```python
from build123d import *

# Parameters (mm, degrees)
SKETCH1_W           = 3.047619048
SKETCH1_H           = 150
SKETCH1_W_2         = 38
SKETCH1_H_2         = 3
BOSS_EXTRUDE1_DEPTH = 15
FILLET1_R           = 10
SKETCH2_R           = 2.5
CUT_EXTRUDE1_DEPTH  = 61
SKETCH3_R           = 2.5
CUT_EXTRUDE2_DEPTH  = 55


with BuildPart() as part:
    # Sketch1 → Boss-Extrude1 (new, symmetric)
    with BuildSketch(Plane.XY):
        with Locations((-20.523809524, 25)):
            Rectangle(SKETCH1_W, SKETCH1_H)
        with Locations((20.523809524, 25)):
            Rectangle(SKETCH1_W, SKETCH1_H)
        with Locations((0, 74.5)):
            Rectangle(SKETCH1_W_2, SKETCH1_H_2)
        with Locations((0, -28.5)):
            Rectangle(SKETCH1_W_2, SKETCH1_H_2)
    extrude(amount=BOSS_EXTRUDE1_DEPTH, both=True)

    # Fillet1
    fillet1_edges = [part.edges().sort_by_distance(p)[0] for p in [
        (-20.523809524, -50, -15),
        (20.523809524, -50, -15),
        (20.523809524, -50, 15),
        (-20.523809524, -50, 15),
        (-20.523809524, 100, 15),
        (-20.523809524, 100, -15),
        (20.523809524, 100, -15),
        (20.523809524, 100, 15),
    ]]
    fillet(fillet1_edges, radius=FILLET1_R)

    # Sketch2 → Cut-Extrude1 (cut)
    with BuildSketch(Plane(origin=(22.047619048, 0, 0), x_dir=(0, 0, -1), z_dir=(1, 0, 0))):
        with Locations(Location((0, 41.439583657, 0), (0, 0, 90))):
            Circle(SKETCH2_R)
        with Locations(Location((0, -40.747770908, 0), (0, 0, 90))):
            Circle(SKETCH2_R)
    extrude(amount=-CUT_EXTRUDE1_DEPTH, mode=Mode.SUBTRACT)

    # Sketch3 → Cut-Extrude2 (cut)
    with BuildSketch(Plane(origin=(22.047619048, 0, 0), x_dir=(0, 0, -1), z_dir=(1, 0, 0))):
        with Locations(Location((0, 90.824457964, 0), (0, 0, 90))):
            Circle(SKETCH3_R)
    extrude(amount=-CUT_EXTRUDE2_DEPTH, mode=Mode.SUBTRACT)


solid = part.part
```
Build history of the part. All positions in model axes, mm. A direction names the side the tool comes from. Coordinates: 2 decimals unless noted, no trailing zeros. Order: outer loops, then holes, each group sorted by start corner. A loop starts at its lowest first (then second) coordinate and runs counter-clockwise, first axis right, second up. Notation, with made-up numbers: (-34, 29) -> (6, 29) arc R20 cw to (6, 42) -> close; hole circle Ø7 at (67, -23). An arc over 180 degrees is marked (long way). Answer in a Markdown table with one row per item. Add a question column.
Q1. Band-saw the part on A-A, the plane y = 53. List the corners of the cut face in (x, z), then the cut area to 3 significant figures.
Q2. Mould opens along X. For faces 4 (the face through (-20.5, 96.99, 12.15)), 5 (the face through (19, -38, 0)), 6 (the face through (-22.048, 24, 0)), 7 (the face through (0, -30, 0)) say: +X half, -X half, draft (parallel to the pull), parting line (faces both ways), or undercut.
Q3. Band-saw the part on C-C, the plane z = -9.5. List the corners of the cut face in (x, y), then the cut area to 3 significant figures.
Q4. Which spindle directions (+Z, -Z, +X, -X, +Y, -Y) get a long thin tool onto all of the face, cutting with end or side? Do faces 1 (the face through (0, 73, 0)), 2 (the face through (-19, 88, 0)), 3 (the face through (-21, 100, 0)). Say none if no direction does.
Q5. Wall check: line 1 along Y through (x, z) = (18, -6); line 2 along X through (y, z) = (1, 12.5). Give the ranges that are in metal, low to high. Write a range as [from, to].
Q6. Drop flat-ended pins along their axis: pin 1 (4.5 mm diameter, centred on y = 90.82, z = 0, fed in from -X); pin 2 (6 mm diameter, centred on x = 13, z = 6, fed in from -Y). Give the stop position or say it passes through.
Q7. Band-saw the part on D-D, the plane z = 0. Give the number of separate pieces and of enclosed holes in the cut face, then the cut area to 3 significant figures.
Q8. Band-saw the part on B-B, the plane x = -17.5. List the corners of the cut face in (y, z).
Answers follow:
| question | item | result |
|---|---|---|
| 1 | outline | (-22.05, -15) -> (-19, -15) -> (-19, 15) -> (-22.05, 15) -> close; (19, -15) -> (22.05, -15) -> (22.05, 15) -> (19, 15) -> close |
| 1 | area | 183 mm^2 |
| 2 | face 4 | draft |
| 2 | face 5 | undercut |
| 2 | face 6 | -X half |
| 2 | face 7 | undercut |
| 3 | outline | (-22.05, -48.93) -> (-19, -48.93) -> (-19, -30) -> (19, -30) -> (19, -48.93) -> (22.05, -48.93) -> (22.05, 98.93) -> (19, 98.93) -> (19, 76) -> (-19, 76) -> (-19, 98.93) -> (-22.05, 98.93) -> close; hole (-19, -27) -> (19, -27) -> (19, 73) -> (-19, 73) -> close |
| 3 | area | 1,130 mm^2 |
| 4 | face 1 | +Z, -Z |
| 4 | face 2 | +Z, -Z, +Y |
| 4 | face 3 | +Z, -Z, +X, -X, +Y |
| 5 | line 1 | [-30, -27], [73, 76] |
| 5 | line 2 | [-22.05, -19], [19, 22.05] |
| 6 | pin 1 | through |
| 6 | pin 2 | y = -30 |
| 7 | separate pieces | 6 |
| 7 | enclosed holes | 0 |
| 7 | area | 1,050 mm^2 |
| 8 | outline | (-30, -15) -> (-27, -15) -> (-27, 15) -> (-30, 15) -> close; (73, -15) -> (76, -15) -> (76, 15) -> (73, 15) -> close |
